The listing builds one solid part. Answer for the finished solid, in the listing's coordinates (mm). A direction names the side the tool comes from. Round coordinates to 2 decimals unless told otherwise and drop trailing zeros. Write each loop counter-clockwise with the first axis right and the second up, starting at its lowest first coordinate (ties: lowest second). Pieces come first, ordered by that corner, then holes.
Item 1: Each of these flat-tipped pins is pushed along its axis until it touches: pin 1 (0.8 mm diameter, centred on x = 32, y = 1.5, fed in from -Z); pin 2 (7 mm diameter, centred on x = 0, z = 0, fed in from +Y); pin 3 (2 mm diameter, centred on x = -4, y = 2.5, fed in from +Z); pin 4 (2.5 mm diameter, centred on x = 22.5, z = -6.7, fed in from +Y). Where does it stop, or does it pass through?
Item 2: Find section C-C on x = 17.5. Give the vertices of the cut face in (y, z).
Item 3: Find section B-B on x = 31.5. Give the vertices of the cut face in (y, z), then the cut area to 3 significant figures.
Item 4: Find section A-A on z = 0. Give the number of separate pieces and of enclosed holes in the cut face, then the cut area to 3 significant figures.
Item 5: Find section D-D on z = -6.7. Give the vertices of the cut face in (x, y), then the cut area to 3 significant figures.
Item 6: For a pull along Z with two mould halves and no side action, classify faces 1 (the face through (4, 2.5, 6)), 2 (the face through (32.79, 1.23, -6.87)), 3 (the face through (8.601, 1.232, 12.115)), 4 (the face through (8.3, 1.23, -12.05)) as +Z half, -Z half, draft (parallel to the pull), parting line (faces both ways), or undercut.
Item 7: A tool of negligible diameter and unlimited length cuts with its end or side. For faces 5 (the face through (35, 1, 0)), 6 (the face through (4, 3.5, 1)), 7 (the face through (-1.802, 3.24, -5.723)), 8 (the face through (24.4, 1.23, -2.13)), from which of +Z, -Z, +X, -X, +Y, -Y can it reach the whole face along a straight path? Write none if from no direction.
Item 8: Find the intervals of material crossed by probe 1 along X at (y, z) = (3.95, 0); probe 2 along Y at (x, z) = (23, 10); probe 3 along X at (y, z) = (1.05, 0.75), in increasing order.
```python
from build123d import *

# Parameters (mm, degrees)
SKETCH1_R           = 1.3
SKETCH1_R_2         = 4.5
SKETCH1_R_3         = 1
BOSS_EXTRUDE1_DEPTH = 2.5
SKETCH3_R           = 6
SKETCH3_R_2         = 3.75
BOSS_EXTRUDE2_DEPTH = 2
SKETCH4_R           = 4.5
SKETCH4_R_2         = 3.75
CUT_EXTRUDE1_DEPTH  = 1
CHAMFER1_SIZE       = 0.5


with BuildPart() as part:
    # Sketch1 → Boss-Extrude1 (new body)
    with BuildSketch(Plane(origin=(0, 0, 0), x_dir=(1, 0, 0), z_dir=(0, 1, 0))):
        with BuildLine():
            Line((35, 9.7), (35, -9.7))
            Line((35, -9.7), (28.656580513, -9.7))
            ThreePointArc((28.656580513, -9.7), (28.032756183, -9.799778117), (27.471175871, -10.089156794))
            Line((27.471175871, -10.089156794), (22.667160445, -13.62438739))
            ThreePointArc((22.667160445, -13.62438739), (20.936486005, -14.401466515), (19.039367435, -14.396259626))
            Line((19.039367435, -14.396259626), (-2.134739034, -9.769487666))
            ThreePointArc((-2.134739034, -9.769487666), (-2.213274492, -9.751995489), (-2.291666667, -9.733871989))
            Line((-2.291666667, -9.733871989), (-25.03125, -4.380242395))
            ThreePointArc((-25.03125, -4.380242395), (-28.5, 0), (-25.03125, 4.380242395))
            Line((-25.03125, 4.380242395), (-2.291666667, 9.733871989))
            ThreePointArc((-2.291666667, 9.733871989), (-2.213276651, 9.751994999), (-2.13474336, 9.769486721))
            Line((-2.13474336, 9.769486721), (19.039365488, 14.396269024))
            ThreePointArc((19.039365488, 14.396269024), (20.936487661, 14.401475987), (22.667164776, 13.624394026))
            Line((22.667164776, 13.624394026), (27.47117527, 10.089158211))
            ThreePointArc((27.47117527, 10.089158211), (28.032756372, 9.799778489), (28.656581837, 9.7))
            Line((28.656581837, 9.7), (35, 9.7))
        make_face()
        with Locations(Location((31.5, 6.7, 0), (0, 0, 270))):
            Circle(SKETCH1_R, mode=Mode.SUBTRACT)
        with Locations(Location((31.5, -6.7, 0), (0, 0, 270))):
            Circle(SKETCH1_R, mode=Mode.SUBTRACT)
        with Locations(Location((20, 10, 0), (0, 0, 270))):
            Circle(SKETCH1_R, mode=Mode.SUBTRACT)
        with Locations(Location((20, -9.999990176, 0), (0, 0, 270))):
            Circle(SKETCH1_R, mode=Mode.SUBTRACT)
        with Locations(Location((0, 0, 0), (0, 0, 270))):
            Circle(SKETCH1_R_2, mode=Mode.SUBTRACT)
        with Locations(Location((-24, 0, 0), (0, 0, 270))):
            Circle(SKETCH1_R, mode=Mode.SUBTRACT)
        with Locations(Location((22.5, -6.7, 0), (0, 0, 270))):
            Circle(SKETCH1_R_3, mode=Mode.SUBTRACT)
        with Locations(Location((22.5, 6.7, 0), (0, 0, 270))):
            Circle(SKETCH1_R_3, mode=Mode.SUBTRACT)
        with BuildLine():
            Line((9.772066478, 8.276878442), (12.216286037, 8.810968065))
            ThreePointArc((12.216286037, 8.810968065), (13.559618748, 8.634777191), (14.482426032, 7.642803041))
            ThreePointArc((14.482426032, 7.642803041), (16.274630398, 5.296637232), (18.968838896, 4.089271891))
            ThreePointArc((18.968838896, 4.089271891), (19.472295347, 3.930738723), (19.916745685, 3.646019459))
            ThreePointArc((19.916745685, 3.646019459), (21.124485944, 2.943943413), (22.5, 2.7))
            Line((22.5, 2.7), (23, 2.7))
            ThreePointArc((23, 2.7), (24.414213562, 2.114213562), (25, 0.7))
            Line((25, 0.7), (25, -0.7))
            ThreePointArc((25, -0.7), (24.414213562, -2.114213562), (23, -2.7))
            Line((23, -2.7), (22.5, -2.7))
            ThreePointArc((22.5, -2.7), (21.124485854, -2.943943446), (19.916745538, -3.646019583))
            ThreePointArc((19.916745538, -3.646019583), (19.472295389, -3.930738787), (18.968839153, -4.089271995))
            ThreePointArc((18.968839153, -4.089271995), (16.274635438, -5.296635948), (14.482434575, -7.642798226))
            ThreePointArc((14.482434575, -7.642798226), (13.559627706, -8.634772461), (12.216295281, -8.810963823))
            Line((12.216295281, -8.810963823), (9.772070143, -8.276874115))
            ThreePointArc((9.772070143, -8.276874115), (8.357168863, -7.102458424), (8.499181625, -5.269147152))
            ThreePointArc((8.499181625, -5.269147152), (10, 2.214e-06), (8.499179292, 5.269150915))
            ThreePointArc((8.499179292, 5.269150915), (8.357165718, 7.102462125), (9.772066478, 8.276878442))
        make_face(mode=Mode.SUBTRACT)
        with BuildLine():
            Line((-17.912878788, -1.946774398), (-12.387619024, -3.247598329))
            ThreePointArc((-12.387619024, -3.247598329), (-10.604369925, -2.799022253), (-9.941071409, -1.084019943))
            ThreePointArc((-9.941071409, -1.084019943), (-10, 0), (-9.941071409, 1.084019943))
            ThreePointArc((-9.941071409, 1.084019943), (-10.604369925, 2.799022253), (-12.387619024, 3.247598329))
            Line((-12.387619024, 3.247598329), (-17.912878788, 1.946774398))
            ThreePointArc((-17.912878788, 1.946774398), (-19.454545455, 0), (-17.912878788, -1.946774398))
        make_face(mode=Mode.SUBTRACT)
    extrude(amount=BOSS_EXTRUDE1_DEPTH)

    # Sketch3 → Boss-Extrude2 (add)
    with BuildSketch(Plane(origin=(0, 2.5, 0), x_dir=(1, 0, 0), z_dir=(0, 1, 0))):
        with Locations(Location((0, 0, 0), (0, 0, 90))):
            Circle(SKETCH3_R)
        with Locations(Location((0, 0, 0), (0, 0, 270))):
            Circle(SKETCH3_R_2, mode=Mode.SUBTRACT)
    extrude(amount=BOSS_EXTRUDE2_DEPTH)

    # Sketch4 → Cut-Extrude1 (cut)
    with BuildSketch(Plane.XZ.offset(-2.5)):
        with Locations(Location((0, 0, 0), (0, 0, 270))):
            Circle(SKETCH4_R)
        with Locations(Location((0, 0, 0), (0, 0, 270))):
            Circle(SKETCH4_R_2, mode=Mode.SUBTRACT)
    extrude(amount=-CUT_EXTRUDE1_DEPTH, mode=Mode.SUBTRACT)

    # Chamfer1
    chamfer1_edges = [part.edges().sort_by_distance(p)[0] for p in [
        (0, 4.5, 6),
    ]]
    chamfer(chamfer1_edges, length=CHAMFER1_SIZE)


solid = part.part
```
Check values:
1. pin 1: stops at z = -9.7
1. pin 2: passes through
1. pin 3: stops at z = 9.57
1. pin 4: stops at y = 2.5
2. outline: (0, -14.06) - (2.5, -14.06) - (2.5, -4.55) - (0, -4.55) - close; (0, 4.55) - (2.5, 4.55) - (2.5, 14.06) - (0, 14.06) - close
3. outline: (0, -9.7) - (2.5, -9.7) - (2.5, -8) - (0, -8) - close; (0, -5.4) - (2.5, -5.4) - (2.5, 5.4) - (0, 5.4) - close; (0, 8) - (2.5, 8) - (2.5, 9.7) - (0, 9.7) - close
3. area: 35.5 mm2
4. separate pieces: 5
4. enclosed holes: 0
4. area: 75.9 mm2
5. outline: (-15.18, 0) - (8.23, 0) - (8.23, 2.5) - (-15.18, 2.5) - close; (14.99, 0) - (21.5, 0) - (21.5, 2.5) - (14.99, 2.5) - close; (23.5, 0) - (30.2, 0) - (30.2, 2.5) - (23.5, 2.5) - close; (32.8, 0) - (35, 0) - (35, 2.5) - (32.8, 2.5) - close
5. area: 97.1 mm2
6. face 1: draft
6. face 2: undercut
6. face 3: +Z half
6. face 4: -Z half
7. face 5: +Z, -Z, +X, +Y, -Y
7. face 6: -Y
7. face 7: +Y
7. face 8: +Y, -Y
8. probe 1: x = -6 to -3.75, 3.75 to 6
8. probe 2: y = 0 to 2.5
8. probe 3: x = -28.44 to -25.06, -22.94 to -19.31, -9.97 to -4.44, 4.44 to 9.97, 25 to 35
